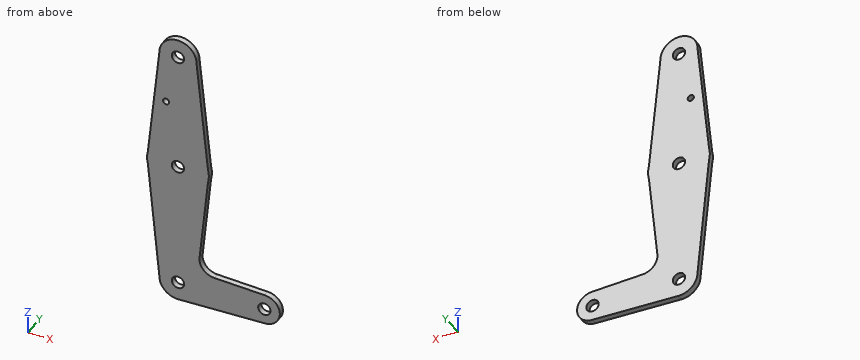
```python
from build123d import *

# Parameters (mm, degrees)
F0_R     = 1.5875
F0_R_2   = 3.175
F1_DEPTH = 3.048


with BuildPart() as f1:
    # F0 (on Front) → F1 (new body)
    with BuildSketch(Plane.XZ):
        with BuildLine():
            Line((15.442731, 36.907912), (9.525, 95.04018))
            ThreePointArc((9.525, 95.04018), (0, 85.51518), (-9.525, 95.04018))
            Line((-9.525, 95.04018), (-15.442731, 36.907912))
            ThreePointArc((-15.442731, 36.907912), (0, 49.103551), (15.442731, 36.907912))
        make_face()
        with Locations((-6.082257, 68.06538)):
            Circle(F0_R, mode=Mode.SUBTRACT)
        with BuildLine():
            ThreePointArc((-9.525, 95.04018), (0, 85.51518), (9.525, 95.04018))
            ThreePointArc((9.525, 95.04018), (0, 104.56518), (-9.525, 95.04018))
        make_face()
        with Locations((0, 95.04018)):
            Circle(F0_R_2, mode=Mode.SUBTRACT)
        with BuildLine():
            ThreePointArc((15.875, 33.228551), (15.766562, 35.080885), (15.442731, 36.907912))
            ThreePointArc((15.442731, 36.907912), (0, 49.103551), (-15.442731, 36.907912))
            ThreePointArc((-15.442731, 36.907912), (-15.875, 33.228551), (-15.442731, 29.549191))
            ThreePointArc((-15.442731, 29.549191), (0, 17.353551), (15.442731, 29.549191))
            ThreePointArc((15.442731, 29.549191), (15.766562, 31.376218), (15.875, 33.228551))
        make_face()
        with Locations((0, 33.228551)):
            Circle(F0_R_2, mode=Mode.SUBTRACT)
        with BuildLine():
            ThreePointArc((9.525, -31.95982), (0, -22.43482), (-9.525, -31.95982))
            ThreePointArc((-9.525, -31.95982), (-6.735192, -38.695012), (0, -41.48482))
            Line((0, -41.48482), (0.67949, -41.460552))
            ThreePointArc((0.67949, -41.460552), (6.97129, -38.450331), (9.525, -31.95982))
        make_face()
        with Locations((0, -31.95982)):
            Circle(F0_R_2, mode=Mode.SUBTRACT)
        with BuildLine():
            ThreePointArc((52.3875, -31.95982), (50.06266, -26.347159), (44.45, -24.02232))
            ThreePointArc((44.45, -24.02232), (36.5125, -31.95982), (44.45, -39.89732))
            ThreePointArc((44.45, -39.89732), (50.06266, -37.57248), (52.3875, -31.95982))
        make_face()
        with Locations((44.45, -31.95982)):
            Circle(F0_R_2, mode=Mode.SUBTRACT)
        with BuildLine():
            ThreePointArc((15.442731, 29.549191), (0, 17.353551), (-15.442731, 29.549191))
            Line((-15.442731, 29.549191), (-9.525, -31.95982))
            ThreePointArc((-9.525, -31.95982), (0, -22.43482), (9.525, -31.95982))
            ThreePointArc((9.525, -31.95982), (6.97129, -38.450331), (0.67949, -41.460552))
            Line((0.67949, -41.460552), (44.45, -39.89732))
            ThreePointArc((44.45, -39.89732), (36.5125, -31.95982), (44.45, -24.02232))
            Line((44.45, -24.02232), (18.711782, -23.103097))
            ThreePointArc((18.711782, -23.103097), (13.018458, -20.39405), (11.096139, -14.389255))
            Line((11.096139, -14.389255), (15.442731, 29.549191))
        make_face()
    extrude(amount=F1_DEPTH)


solid = f1.part
```
Could you check a few things on this model? Use its own coordinates, in mm. Coordinates: 2 decimals unless noted, no trailing zeros. Write each loop counter-clockwise with the first axis right and the second up, starting at its lowest first coordinate (ties: lowest second). Pieces come first, ordered by that corner, then holes. Notation, with made-up numbers: M 68,83.5 L 112,83.5 A27 ccw 112,117.5 Z; hole C 9.25,-19.5 d9. An arc over 180 degrees is marked long. Answer as CSV lines item,"result". Start each with the question number.
1) I want a section at A-A, the plane y = -1.5. Give the number of separate pieces and of enclosed holes in the cut face, and give its area (3 significant figures).
2) I want a section at C-C, the plane z = 39.5. Please give me the cut outline in (x, y), and give its area (3 significant figures).
3) Please list where these lines run through material, in increasing order: line 1 (Z direction, x = 44, y = -2.45); line 2 (Z direction, x = 1.5, y = -2.25); line 3 (Z direction, x = -7, y = -1.4). Write a range as from..to.
4) I want a section at B-B, the plane z = 3. Please give me the cut outline in (x, y).
Data:
1,separate pieces,"1"
1,enclosed holes,"5"
1,area,"4,090 mm^2"
2,outline,"M -15.18,-3.05 L 15.18,-3.05 L 15.18,0 L -15.18,0 Z"
2,area,"92.5 mm^2"
3,line 1,"z = -39.91..-35.1, -28.82..-24.01"
3,line 2,"z = -41.43..-34.76, -29.16..30.43, 36.03..92.24, 97.84..104.45"
3,line 3,"z = -38.42..66.77, 69.36..101.5"
4,outline,"M -12.89,-3.05 L 12.82,-3.05 L 12.82,0 L -12.89,0 Z"
